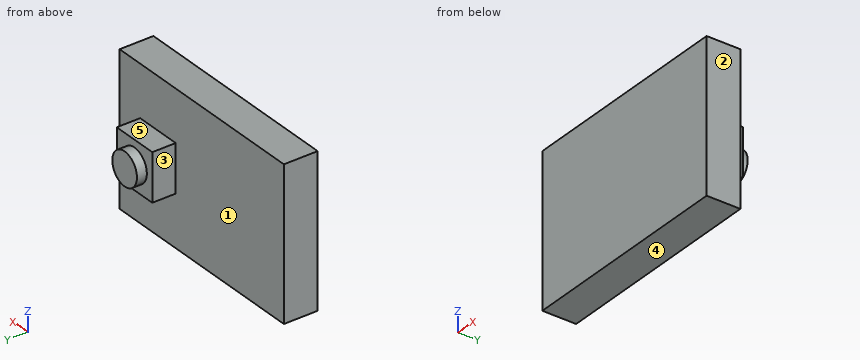
```python
from build123d import *

# Parameters (mm, degrees)
SKETCH_1_W      = 40
SKETCH_1_H      = 27.3
EXTRUDE_1_DEPTH = 6.15
EXTRUDE_START   = -6.15
SKETCH_2_W      = 8.65
SKETCH_2_H      = 8.65
EXTRUDE_2_DEPTH = 10.4
SKETCH_3_R      = 3
EXTRUDE_3_DEPTH = 1.8


with BuildPart() as part:
    # 草图1 → 凸台-拉伸1 (new body)
    with BuildSketch(Plane(origin=(0, 0, 0), x_dir=(1, 0, 0), z_dir=(0, 1, 0))):
        Rectangle(SKETCH_1_W, SKETCH_1_H)
    extrude(amount=EXTRUDE_1_DEPTH)

    # 草图2 → 凸台-拉伸2 (add)
    with BuildSketch(Plane(origin=(0, 6.15, 0), x_dir=(1, 0, 0), z_dir=(0, 1, 0)).offset(EXTRUDE_START)):
        with Locations((10.675, 0)):
            Rectangle(SKETCH_2_W, SKETCH_2_H)
    extrude(amount=EXTRUDE_2_DEPTH)

    # 草图3 → 凸台-拉伸3 (add)
    with BuildSketch(Plane(origin=(0, 10.4, 0), x_dir=(1, 0, 0), z_dir=(0, 1, 0))):
        with Locations(Location((10.675, 0, 0), (0, 0, 270))):
            Circle(SKETCH_3_R)
    extrude(amount=EXTRUDE_3_DEPTH)


solid = part.part
```
Geometry check sheet. Reference: the model listing, model coordinates, mm. Face numbers are marked on the shaded views. A direction names the side the tool comes from. Coordinates: 2 decimals unless noted, no trailing zeros. Loops run counter-clockwise (first coordinate to the right, second up) from the corner with the lowest first, then second, coordinate; pieces in that order, holes last.
Item 1: Release check for a two-part mould opening along X. For the marked faces 1, 2 and 3 record: released by +X, released by -X, zero draft, split by the parting line, or undercut.
Item 2: Access from +Z, -Z, +X, -X, +Y, -Y to the whole of each face (thin tool, end or side, straight path). Record for the marked faces 4 and 5.
Item 3: Sectioned sample at A-A, the plane z = 0. Record the boundary of the cut face in (x, y) (3 decimals), then the cut area to 3 significant figures.
Item 4: Thickness scan on line 1 (X direction, y = 8, z = 2.5); line 2 (Y direction, x = 0, z = -7.5); line 3 (X direction, y = 11.75, z = -2). Record the ranges inside material, lowest first.
Item 5: Sectioned sample at B-B, the plane x = -7. Record the boundary of the cut face in (y, z), then the cut area to 3 significant figures.
Item 6: Go/stop test with flat-tipped pins: pin 1 Ø12 at (x, z) = (0, 8) entering from +Y; pin 2 Ø10 at (x, z) = (6, -8) entering from -Y; pin 3 Ø2 at (x, y) = (12, 9) entering from -Z (3 decimals). Record where each tip stops, or that it passes through.
Item 7: Sectioned sample at C-C, the plane y = 9.75. Record the boundary of the cut face in (x, z) (3 decimals), then the cut area to 3 significant figures.
Check result:
1. face 1: zero draft
1. face 2: released by +X
1. face 3: released by -X
2. face 4: -Z, +X, -X, +Y, -Y
2. face 5: +Z, +X, -X, +Y
3. outline: (-20, 0) - (20, 0) - (20, 6.15) - (15, 6.15) - (15, 10.4) - (13.675, 10.4) - (13.675, 12.2) - (7.675, 12.2) - (7.675, 10.4) - (6.35, 10.4) - (6.35, 6.15) - (-20, 6.15) - close
3. area: 294 mm2
4. line 1: x = 6.35 to 15
4. line 2: y = 0 to 6.15
4. line 3: x = 8.44 to 12.91
5. outline: (0, -13.65) - (6.15, -13.65) - (6.15, 13.65) - (0, 13.65) - close
5. area: 168 mm2
6. pin 1: stops at y = 6.15
6. pin 2: stops at y = 0
6. pin 3: stops at z = -4.325
7. outline: (6.35, -4.325) - (15, -4.325) - (15, 4.325) - (6.35, 4.325) - close
7. area: 74.8 mm2
